Could you check a few things on this model? Use its own coordinates, in mm. Face numbers are marked on the shaded views. A direction names the side the tool comes from. Give positions to 0.01 mm unless a question says otherwise; leave off trailing zeros. Write each loop counter-clockwise with the first axis right and the second up, starting at its lowest first coordinate (ties: lowest second). Pieces come first, ordered by that corner, then holes. Notation, with made-up numbers: (88.5, 30) - (121.5, 30) arc R24 cw to (121.5, 48) - close; hole circle Ø11 at (20, 69). An arc over 180 degrees is marked (long way). Write item = value, one per line.
from build123d import *

# Parameters (mm, degrees)
F0_R     = 1.1684
F1_DEPTH = 1.1811
F3_DEPTH = 4.953
F5_DEPTH = 3.4798
F7_DEPTH = 4.4069


with BuildPart() as f1:
    # F0 (on Top) → F1 (new body, symmetric)
    with BuildSketch(Plane.XY):
        with BuildLine():
            Line((16.6497, 4.4577), (-16.6497, 4.4577))
            ThreePointArc((-16.6497, 4.4577), (-17.763252, 3.996452), (-18.2245, 2.8829))
            Line((-18.2245, 2.8829), (-18.2245, -2.8829))
            ThreePointArc((-18.2245, -2.8829), (-17.763252, -3.996452), (-16.6497, -4.4577))
            Line((-16.6497, -4.4577), (16.6497, -4.4577))
            ThreePointArc((16.6497, -4.4577), (17.763252, -3.996452), (18.2245, -2.8829))
            Line((18.2245, -2.8829), (18.2245, 2.8829))
            ThreePointArc((18.2245, 2.8829), (17.763252, 3.996452), (16.6497, 4.4577))
        make_face()
        with Locations((-15.4305, 0)):
            Circle(F0_R, mode=Mode.SUBTRACT)
        with Locations((15.4305, 0)):
            Circle(F0_R, mode=Mode.SUBTRACT)
    extrude(amount=F1_DEPTH, both=True)

    # F2 (on face) → F3 (join)
    with BuildSketch(Plane.XY.offset(1.1811)):
        with BuildLine():
            Line((-11.96962, -3.7592), (11.971078, -3.7592))
            ThreePointArc((11.971078, -3.7592), (13.327971, -2.983671), (13.348429, -1.420922))
            Line((13.348429, -1.420922), (10.926763, 2.947878))
            ThreePointArc((10.926763, 2.947878), (10.348684, 3.541294), (9.549412, 3.7592))
            Line((9.549412, 3.7592), (-9.547955, 3.7592))
            ThreePointArc((-9.547955, 3.7592), (-10.347226, 3.541294), (-10.925306, 2.947878))
            Line((-10.925306, 2.947878), (-13.346971, -1.420922))
            ThreePointArc((-13.346971, -1.420922), (-13.326514, -2.983671), (-11.96962, -3.7592))
        make_face()
    extrude(amount=F3_DEPTH)

    # F4 (on face) → F5 (join)
    with BuildSketch(Plane(origin=(0, 0, -1.1811), x_dir=(1, 0, 0), z_dir=(0, 0, -1))):
        with BuildLine():
            Line((12.7, 2.8956), (-12.7, 2.8956))
            ThreePointArc((-12.7, 2.8956), (-13.149013, 2.709613), (-13.335, 2.2606))
            Line((-13.335, 2.2606), (-13.335, -2.2606))
            ThreePointArc((-13.335, -2.2606), (-13.149013, -2.709613), (-12.7, -2.8956))
            Line((-12.7, -2.8956), (12.7, -2.8956))
            ThreePointArc((12.7, -2.8956), (13.149013, -2.709613), (13.335, -2.2606))
            Line((13.335, -2.2606), (13.335, 2.2606))
            ThreePointArc((13.335, 2.2606), (13.149013, 2.709613), (12.7, 2.8956))
        make_face()
    extrude(amount=F5_DEPTH)

    # F6 (on face) → F7 (cut)
    with BuildSketch(Plane.XY.offset(6.1341)):
        with BuildLine():
            Line((9.36239, 3.4417), (-9.360933, 3.4417))
            ThreePointArc((-9.360933, 3.4417), (-10.160204, 3.223794), (-10.738284, 2.630378))
            Line((-10.738284, 2.630378), (-13.058827, -1.555992))
            ThreePointArc((-13.058827, -1.555992), (-13.042329, -2.816274), (-11.94806, -3.4417))
            Line((-11.94806, -3.4417), (11.949517, -3.4417))
            ThreePointArc((11.949517, -3.4417), (13.043786, -2.816274), (13.060284, -1.555992))
            Line((13.060284, -1.555992), (10.739742, 2.630378))
            ThreePointArc((10.739742, 2.630378), (10.161662, 3.223794), (9.36239, 3.4417))
        make_face()
    extrude(amount=-F7_DEPTH, mode=Mode.SUBTRACT)


solid = f1.part
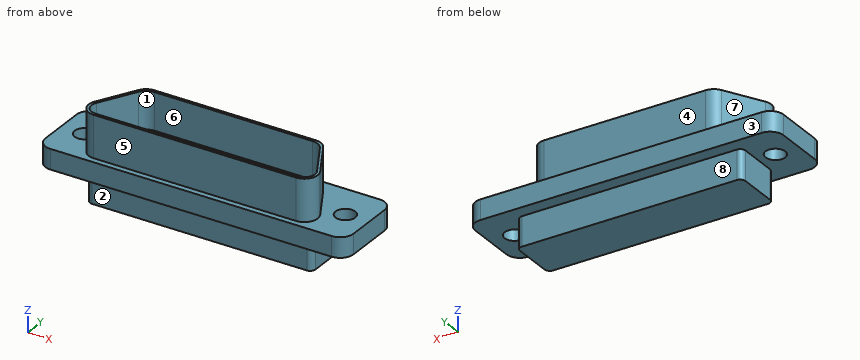
1. For pin 1 (4 mm diameter, centred on x = 4, z = -2.5, fed in from -Y); pin 2 (1 mm diameter, centred on x = -10, z = 3.5, fed in from -Y); pin 3 (1.5 mm diameter, centred on x = -4.5, z = 3.5, fed in from +Y); pin 4 (4 mm diameter, centred on x = 3.5, z = -3.5, fed in from +Y), each with a flat end and sliding along its axis, tell me the tip position at first contact or that it passes through.
Filled sheet:
pin_1 = -4.46
pin_2 = -3.76
pin_3 = 3.76
pin_4 = 2.9
2. I need wall thicknesses on line 1 (Y direction, x = 5.5, z = 2); line 2 (Y direction, x = -6, z = -3.25); line 3 (Z direction, x = 7, y = -2). Which ranges of each line are inside material? Lowest first, please.
Filled sheet:
line_1 = -3.76 to -3.44, 3.44 to 3.76
line_2 = -2.9 to 2.9
line_3 = -4.66 to 1.73
3. Which directions (+Z, -Z, +X, -X, +Y, -Y) give clear straight access to the entire face, cutting with the end or side of a thin tool? Please do the marked faces 4, 5, 6, 7 and 8.
Filled sheet:
face_4 = +Z, +X, -X, +Y
face_5 = +Z, +X, -X, -Y
face_6 = +Z
face_7 = +Z, -X, +Y
face_8 = -Z, +X, -X, +Y
4. If we section it at B-B, the plane z = -0.25: Please give me the cut outline in (x, y), and give its area (3 significant figures).
Filled sheet:
outline = (-18.22, -2.88) arc R1.57 ccw to (-16.65, -4.46) - (16.65, -4.46) arc R1.57 ccw to (18.22, -2.88) - (18.22, 2.88) arc R1.57 ccw to (16.65, 4.46) - (-16.65, 4.46) arc R1.57 ccw to (-18.22, 2.88) - close; hole circle Ø2.34 at (-15.43, 0); hole circle Ø2.34 at (15.43, 0)
area = 314 mm2
5. If we section it at C-C, the plane z = 4.25: Please give me the cut outline in (x, y), and give its area (3 significant figures).
Filled sheet:
outline = (-13.35, -1.42) arc R1.57 ccw to (-11.97, -3.76) - (11.97, -3.76) arc R1.57 ccw to (13.35, -1.42) - (10.93, 2.95) arc R1.57 ccw to (9.55, 3.76) - (-9.55, 3.76) arc R1.57 ccw to (-10.93, 2.95) - close; hole (-13.06, -1.56) arc R1.27 ccw to (-11.95, -3.44) - (11.95, -3.44) arc R1.27 ccw to (13.06, -1.56) - (10.74, 2.63) arc R1.57 ccw to (9.36, 3.44) - (-9.36, 3.44) arc R1.57 ccw to (-10.74, 2.63) - close
area = 19.8 mm2
6. If we section it at A-A, the plane y = 0: Count the separate pieces of the cut face and the enclosed holes in it, and give its area (3 significant figures).
Filled sheet:
separate_pieces = 3
enclosed_holes = 0
area = 185 mm2
7. If we section it at D-D, the plane x = 2: Please give me the cut outline in (y, z), and give its area (3 significant figures).
Filled sheet:
outline = (-4.46, -1.18) - (-2.9, -1.18) - (-2.9, -4.66) - (2.9, -4.66) - (2.9, -1.18) - (4.46, -1.18) - (4.46, 1.18) - (3.76, 1.18) - (3.76, 6.13) - (3.44, 6.13) - (3.44, 1.73) - (-3.44, 1.73) - (-3.44, 6.13) - (-3.76, 6.13) - (-3.76, 1.18) - (-4.46, 1.18) - close
area = 48.1 mm2
8. Thinking about a two-plate mould opening in Y: for the marked faces 1, 2 and 3, which applies, pulls with the +Y half, pulls with the -Y half, needs draft (parallel to the pull), parting line crosses it, or undercut?
Filled sheet:
face_1 = undercut
face_2 = pulls with the -Y half
face_3 = pulls with the +Y half
